Autodesk Inventor part; units mm, degrees
ref_plane "YZ Plane" through (0, 0, 0) normal (1, 0, 0) x (0, 1, 0)
ref_plane "XZ Plane" through (0, 0, 0) normal (0, 1, 0) x (-1, 0, 0)
ref_plane "XY Plane" through (0, 0, 0) normal (0, 0, 1) x (1, 0, 0)
sketch "Sketch4" plane through (0, 0, 0) normal (0, 0, 1) x (1, 0, 0)
  line L0 (-2.4, 0) -> (4, 0)
  line L1 (0, 0) -> (-2.4, 0)
  line L2 (0, 2.8) -> (0, 1.97)
  line L3 (0.5, 1.47) -> (0.5, 1.47)
  line L4 (0.5, 1.47) -> (1, 1.5)
  arc A0 (0, 1.97) -> (0.5, 1.47) centre (0.5, 1.97) ccw
  line L5 (-2.4, 0) -> (-2.4, 1.5)
  line L6 (0, 2.8) -> (-1.4761, 2.8)
  arc A1 (-1.4761, 2.8) -> (-2.4, 1.5) centre (2.0854, -0.7093) ccw
  line L7 (1, 1.5) -> (4, 1.5)
  line L8 (4, 1.5) -> (4, 0)
  point P0 (0, 1.47)
  dimension "d71" = 0.5
  dimension "d72" = 4
  dimension "d74" = 0.5
  dimension "d75" = 2.94
  dimension "d78" = 3
  dimension "d82" = 5
  dimension "d83" = 2.4
  dimension "d84" = 5.6
  dimension "d104" = 3
  dimension "d105" = 3
revolve "Revolution7" add sketch "Sketch4" angle 360 about axis through (-2.4, 0, 0) along (1, 0, 0)
sketch "Sketch5" plane through (-2.4, 0, 0) normal (-1, 0, 0) x (0, 0, 1)
  circle A0 centre (0, 0) radius 1.4 construction
  circle A1 centre (0, 0) radius 0.98 construction
  line L0 (0, 0) -> (-0.8487, 0.49)
  line L1 (0, 0) -> (-0.8487, -0.49)
  line L2 (-1.8008, 0) -> (1.7887, 0)
  line L3 (-1.4, 0) -> (-0.8487, -0.49)
  line L4 (-1.4, 0) -> (-0.8487, 0.49)
  point P0 (0, 0)
  dimension "d88" = 2.8
  dimension "d89" = 1.96
  dimension "d90" = 30
  dimension "d91" = 30
extrude "Extrusion1" cut sketch "Sketch5" against normal blind 1.27
pattern_circular "Circular Pattern1" count 6 over 360 about axis through (-10, 0, 0) along (1, 0, 0) of "Extrusion1"
fillet "Fillet1" radius 0.28 12 edges at (-1.765, -1.2124, -0.7) (-1.765, -0.49, -0.8487) (-1.765, -0.98, 0) (-1.765, -1.2124, 0.7) (-1.765, -0.49, 0.8487) (-1.765, 0, 1.4) (-1.765, 0.98, 0) (-1.765, 1.2124, 0.7) (-1.765, 0.49, 0.8487) (-1.765, 0.49, -0.8487) (-1.765, 0, -1.4) (-1.765, 1.2124, -0.7)
thread "Thread7"
properties part number "Šroub s válcovou hlavou a šestiramennou drážkou ISO 14583 - M3 x 4 - 4.8" material "Ocel"
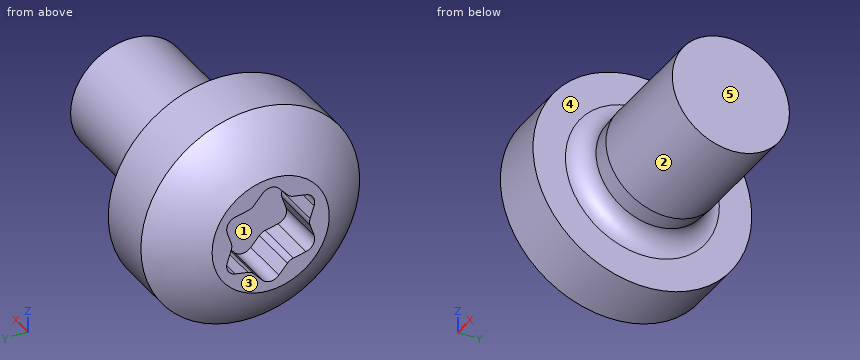
Input: part model. Units: mm. Frame: model coordinates. Face numbers are marked on the shaded views. A direction names the side the tool comes from. Coordinates: 2 decimals unless noted, no trailing zeros. Write each loop counter-clockwise with the first axis right and the second up, starting at its lowest first coordinate (ties: lowest second). Pieces come first, ordered by that corner, then holes.
1) Section A-A on x = 1.75. Output: boundary loops of the cut face in (y, z), and give its area (3 significant figures).
2) Pin query (flat end, axial travel): pin 1 Ø2 at (y, z) = (1, 0.5) entering from -X; pin 2 Ø1.1 at (y, z) = (0, -0.5) entering from -X; pin 3 Ø1 at (x, y) = (2.5, 1) entering from +Z. Return the tip coordinate at first contact, or that it passes through.
3) Material intervals for line 1 along Y through (x, z) = (-1.75, -1); line 2 along Z through (x, y) = (-1.5, -0.3); line 3 along Z through (x, y) = (0.25, 0.2), sorted ascending.
4) Set-up query: the marked faces 4 and 5. Return all of +Z, -Z, +X, -X, +Y, -Y with unobstructed straight access to the full face (end or side cutting, diameter ignored); none if empty.
5) Mould query, pull axis Y, two halves, no side actions, for the marked faces 1, 2 and 3. Classes: pulls with the +Y half, pulls with the -Y half, needs draft (parallel to the pull), parting line crosses it, or undercut.
6) Section B-B on x = -0.25. Output: boundary loops of the cut face in (y, z).
Check result:
1. outline: circle Ø3 at (0, 0)
1. area: 7.07 mm2
2. pin 1: stops at x = -2.4
2. pin 2: stops at x = -1.13
2. pin 3: stops at z = 1.41
3. line 1: y = -2.29 to -0.36, 0.36 to 2.29
3. line 2: z = -2.76 to -1.06, 1.06 to 2.76
3. line 3: z = -1.52 to 1.52
4. face 4: +X
4. face 5: +Z, -Z, +X, +Y, -Y
5. face 1: undercut
5. face 2: parting line crosses it
5. face 3: needs draft
6. outline: circle Ø5.6 at (0, 0)
